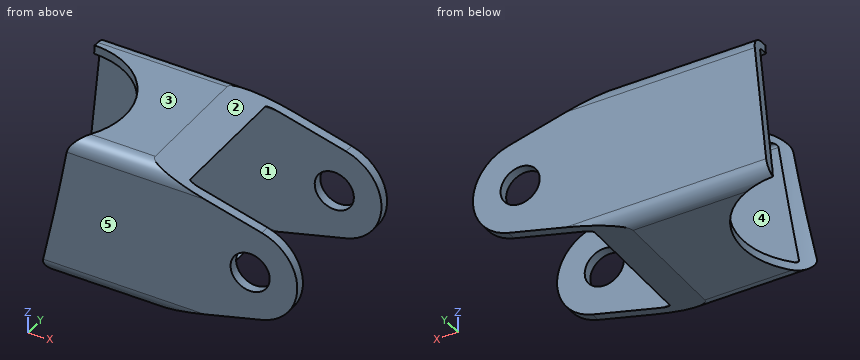
```python
from build123d import *

# Parameters (mm, degrees)
BOSS_EXTRUDE1_DEPTH      = 25.4
BOSS_EXTRUDE1_DEPTH_BACK = 34.925
CUT_EXTRUDE4_DEPTH       = 63.941922635
CUT_EXTRUDE5_DEPTH       = 46.01339384
SKETCH14_R               = 3.2893
CUT_EXTRUDE6_DEPTH       = 46.01339384
CUT_EXTRUDE7_DEPTH       = 56.927898629
CUT_EXTRUDE7_DEPTH_BACK  = 56.927898629
SKETCH15_R               = 12.7
SKETCH17_W               = 59.080455772
SKETCH17_H               = 55.148842709
CUT_EXTRUDE8_DEPTH       = 52.94853237


with BuildPart() as part:
    # Sketch1 → Boss-Extrude1 (new, two sides: drawn at the far end of the back side and taken through both)
    with BuildSketch(Plane(origin=(0, 0, 0), x_dir=(0, 0, -1), z_dir=(1, 0, 0)).offset(-BOSS_EXTRUDE1_DEPTH_BACK)):
        with BuildLine():
            Line((-10.16, 12.7), (10.16, 12.7))
            ThreePointArc((10.16, 12.7), (11.956051224, 11.956051224), (12.7, 10.16))
            Line((12.7, 10.16), (12.7, -10.16))
            ThreePointArc((12.7, -10.16), (11.956051224, -11.956051224), (10.16, -12.7))
            Line((10.16, -12.7), (-10.16, -12.7))
            ThreePointArc((-10.16, -12.7), (-11.956051224, -11.956051224), (-12.7, -10.16))
            Line((-12.7, -10.16), (-12.7, 10.16))
            ThreePointArc((-12.7, 10.16), (-11.956051224, 11.956051224), (-10.16, 12.7))
        make_face()
    extrude(amount=BOSS_EXTRUDE1_DEPTH + BOSS_EXTRUDE1_DEPTH_BACK)

    # Sketch11 → Cut-Extrude4 (cut, through all)
    with BuildSketch(Plane(origin=(25.4, 0, 0), x_dir=(0, 0, -1), z_dir=(1, 0, 0))):
        with BuildLine():
            Line((-10.6045, 11.1125), (10.6045, 11.1125))
            ThreePointArc((10.6045, 11.1125), (10.963710245, 10.963710245), (11.1125, 10.6045))
            Line((11.1125, 10.6045), (11.1125, -10.6045))
            ThreePointArc((11.1125, -10.6045), (10.963710245, -10.963710245), (10.6045, -11.1125))
            Line((10.6045, -11.1125), (-10.6045, -11.1125))
            ThreePointArc((-10.6045, -11.1125), (-10.963710245, -10.963710245), (-11.1125, -10.6045))
            Line((-11.1125, -10.6045), (-11.1125, 10.6045))
            ThreePointArc((-11.1125, 10.6045), (-10.963710245, 10.963710245), (-10.6045, 11.1125))
        make_face()
    extrude(amount=-CUT_EXTRUDE4_DEPTH, mode=Mode.SUBTRACT)

    # Sketch12 → Cut-Extrude5 (cut, through all)
    with BuildSketch(Plane(origin=(0, 12.7, 0), x_dir=(1, 0, 0), z_dir=(0, 1, 0))):
        with BuildLine():
            Line((0, 12.7), (50.8, 12.7))
            Line((50.8, 12.7), (50.8, -12.7))
            Line((50.8, -12.7), (0, -12.7))
            Line((0, -12.7), (19.444424463, -7.686083637))
            ThreePointArc((19.444424463, -7.686083637), (25.4, 0), (19.444424463, 7.686083637))
            Line((19.444424463, 7.686083637), (0, 12.7))
        make_face()
    extrude(amount=-CUT_EXTRUDE5_DEPTH, mode=Mode.SUBTRACT)

    # Sketch14 → Cut-Extrude6 (cut, through all)
    with BuildSketch(Plane(origin=(0, 12.7, 0), x_dir=(1, 0, 0), z_dir=(0, 1, 0))):
        with Locations(Location((17.4625, 0, 0), (0, 0, 270))):
            Circle(SKETCH14_R)
    extrude(amount=-CUT_EXTRUDE6_DEPTH, mode=Mode.SUBTRACT)

    # Sketch15 → Cut-Extrude7 (cut, two sides: drawn at the far end of the back side and taken through both)
    with BuildSketch(Plane(origin=(-21.74366369, -3.432105223, 12.7), x_dir=(-0.9956294808615993, -0.006900458495911936, 0.09313603229582201), z_dir=(-0.09339131029845446, 0.07356465915336342, -0.9929080038374085)).offset(-CUT_EXTRUDE7_DEPTH_BACK)):
        Circle(SKETCH15_R)
    extrude(amount=CUT_EXTRUDE7_DEPTH + CUT_EXTRUDE7_DEPTH_BACK, mode=Mode.SUBTRACT)

    # Sketch17 → Cut-Extrude8 (cut, through all)
    with BuildSketch(Plane(origin=(-22.73705084, 0, 2.138609984), x_dir=(-0.09339131029845445, 0.07356465915336355, -0.9929080038374085), z_dir=(0.9956056474877124, 0, -0.09364504626819836))):
        with Locations((0.199202034, -0.945767637)):
            Rectangle(SKETCH17_W, SKETCH17_H)
    extrude(amount=-CUT_EXTRUDE8_DEPTH, mode=Mode.SUBTRACT)


solid = part.part
```
Source: CAD feature listing. Evaluate the final solid. Frame: model axes, mm. Face numbers are marked on the shaded views. A direction names the side the tool comes from. Round coordinates to 2 decimals unless told otherwise and drop trailing zeros. Write each loop counter-clockwise with the first axis right and the second up, starting at its lowest first coordinate (ties: lowest second). Pieces come first, ordered by that corner, then holes. Notation, with made-up numbers: M 39,50 L 65,50 A24 cw 65,66 Z; hole C -6.5,-28 d4. An arc over 180 degrees is marked long. Use CSV: the item, a comma, the result in double quotes. Start each with the question number.
Q1. Pull-direction query (Y, two-part tool) for the marked faces 3, 4 and 5; classes: +Y half, -Y half, draft (parallel to the pull), parting line (faces both ways), or undercut.
Q2. Access query for the marked faces 1 and 2. Directions: +Z, -Z, +X, -X, +Y, -Y. A direction counts if a zero-diameter tool reaches every point of the face in a straight line with its end or side. Return the directions, or none.
Q3. Line query: line 1 (Y direction, x = 0, z = -2.5); line 2 (Z direction, x = 5.5, y = -3.75). Output: solid intervals per line, ascending. Write a range as from..to.
Q4. Cut plane A-A on x = 15. Output: boundary loops of the cut face in (y, z), plus the area to 3 significant figures.
Q5. First-contact query: P1, Ø4, axis at y = 3.5, z = 9, coming from the -X side; P2, Ø5, axis at y = 2.5, z = 9.5, coming from the +X side; P3, Ø4, axis at x = -19, z = -1, coming from the -Y side. Flat tips, straight axial feed; report the tip coordinate or a pass-through.
Q6. Cut plane B-B on z = -0.5. Count the separate pieces of the cut face and the enclosed holes in it, plus the area to 3 significant figures.
Results found:
1,face 3,"draft"
1,face 4,"undercut"
1,face 5,"-Y half"
2,face 1,"+X, -X"
2,face 2,"+Z, +X, +Y, -Y"
3,line 1,"-12.7..-11.11, 11.11..12.7"
3,line 2,"-11.28..-11.11, 11.11..11.28"
4,outline,"M -12.7,-8.83 L -11.11,-8.83 L -11.11,-2.18 L -12.7,-2.18 Z; M -12.7,2.18 L -11.11,2.18 L -11.11,8.83 L -12.7,8.83 Z; M 11.11,-8.83 L 12.7,-8.83 L 12.7,-2.18 L 11.11,-2.18 Z; M 11.11,2.18 L 12.7,2.18 L 12.7,8.83 L 11.11,8.83 Z"
4,area,"42.2 mm^2"
5,P1,"through"
5,P2,"x = 6.16"
5,P3,"y = 11.11"
6,separate pieces,"4"
6,enclosed holes,"0"
6,area,"119 mm^2"
